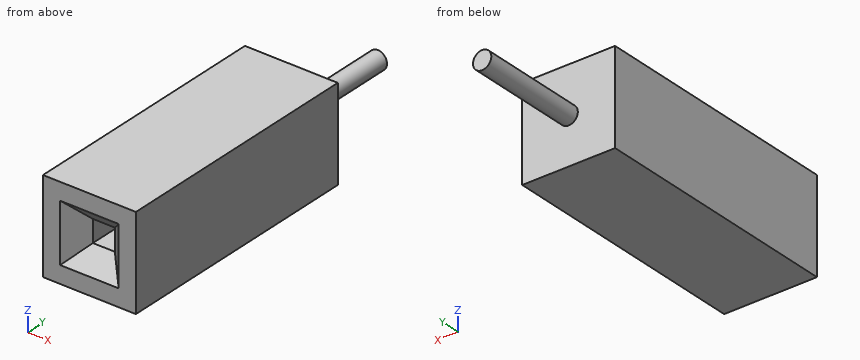
Autodesk Inventor part; units mm, degrees
ref_plane "YZ Plane" through (0, 0, 0) normal (1, 0, 0) x (0, 1, 0)
ref_plane "XZ Plane" through (0, 0, 0) normal (0, 1, 0) x (-1, 0, 0)
ref_plane "XY Plane" through (0, 0, 0) normal (0, 0, 1) x (1, 0, 0)
sketch "Sketch1" plane through (0, 0, 0) normal (0, 1, 0) x (-1, 0, 0)
  line L0 (1.27, -1.27) -> (-1.27, -1.27)
  line L1 (-1.27, -1.27) -> (-1.27, 1.27)
  line L2 (-1.27, 1.27) -> (1.27, 1.27)
  line L3 (1.27, 1.27) -> (1.27, -1.27)
  point P0 (0, 0)
  point P1 (0, -1.27)
  point P2 (1.27, 0)
  dimension "d2" = 2.54
extrude "Extrusion1" add sketch "Sketch1" along normal blind 7
sketch "Sketch6" plane through (0, 7, 0) normal (0, 1, 0) x (1, 0, 0)
  circle A0 centre (0, 0) radius 0.25
  dimension "d19" = 0.5
sketch "Sketch7" plane through (0, 0, 0) normal (0, -1, 0) x (1, 0, 0)
  line L0 (-0.3, 0.3) -> (0.3, 0.3)
  line L1 (0.3, 0.3) -> (0.3, -0.3)
  line L2 (0.3, -0.3) -> (-0.3, -0.3)
  line L3 (-0.3, -0.3) -> (-0.3, 0.3)
  point P0 (0, 0)
  point P1 (0, 0.3)
  point P2 (-0.3, 0)
  dimension "d20" = 0.6
extrude "Extrusion4" cut sketch "Sketch7" against normal blind 5
chamfer "Chamfer1" distance 0.5 angle 45 4 edges at (0, 0, 0.3) (0.3, 0, 0) (0, 0, -0.3) (-0.3, 0, 0)
extrude "Extrusion5" add sketch "Sketch6" along normal blind 3
properties part number "Pin-round-2.54-female"
Build history of the part. All positions in model axes, mm. Coordinates: 2 decimals unless noted, no trailing zeros. Order: outer loops, then holes, each group sorted by start corner. A loop starts at its lowest first (then second) coordinate and runs counter-clockwise, first axis right, second up. Notation, with made-up numbers: (-21, 19) -> (25, 19) arc R17 cw to (25, 43) -> close; hole circle Ø8 at (51.5, -35). An arc over 180 degrees is marked (long way). One line per item, written item: value.
(1) Slice it at B-B, the plane x = 0.6. List the corners of the cut face in (y, z), plus the area to 3 significant figures.
Checked values:
outline: (0, -1.27) -> (7, -1.27) -> (7, 1.27) -> (0, 1.27) -> (0, 0.8) -> (0.2, 0.6) -> (0.2, -0.6) -> (0, -0.8) -> close
area: 17.5 mm2
(2) Drop flat-ended pins along their axis: pin 1 Ø1 at (x, z) = (-1, 1) entering from +Y; pin 2 Ø0.5 at (x, z) = (0, 0) entering from -Y. Give the stop position or say it passes through.
Checked values:
pin 1: y = 7
pin 2: y = 5
(3) Slice it at D-D, the plane x = 0. List the corners of the cut face in (y, z), plus the area to 3 significant figures.
Checked values:
outline: (0, -1.27) -> (7, -1.27) -> (7, -0.25) -> (10, -0.25) -> (10, 0.25) -> (7, 0.25) -> (7, 1.27) -> (0, 1.27) -> (0, 0.8) -> (0.5, 0.3) -> (5, 0.3) -> (5, -0.3) -> (0.5, -0.3) -> (0, -0.8) -> close
area: 16.0 mm2
(4) Probe line 1 (X direction, y = 4, z = -0.15); line 2 (Y direction, x = -0.3, z = -1.05). List the from-to ranges inside material, lowest first. Write a range as [from, to].
Checked values:
line 1: [-1.27, -0.3], [0.3, 1.27]
line 2: [0, 7]
(5) Slice it at C-C, the plane z = 0. List the corners of the cut face in (x, y).
Checked values:
outline: (-1.27, 0) -> (-0.8, 0) -> (-0.3, 0.5) -> (-0.3, 5) -> (0.3, 5) -> (0.3, 0.5) -> (0.8, 0) -> (1.27, 0) -> (1.27, 7) -> (0.25, 7) -> (0.25, 10) -> (-0.25, 10) -> (-0.25, 7) -> (-1.27, 7) -> close
(6) Slice it at A-A, the plane y = 1. List the corners of the cut face in (x, z), plus the area to 3 significant figures.
Checked values:
outline: (-1.27, -1.27) -> (1.27, -1.27) -> (1.27, 1.27) -> (-1.27, 1.27) -> close; hole (-0.3, -0.3) -> (0.3, -0.3) -> (0.3, 0.3) -> (-0.3, 0.3) -> close
area: 6.09 mm2
